from build123d import *

# Parameters (mm, degrees)
CROQUIS1_R              = 2.15
SALIENTE_EXTRUIR1_DEPTH = 320.6


with BuildPart() as part:
    # Croquis1 → Saliente-Extruir1 (new body)
    with BuildSketch(Plane.XY):
        Polygon((20, 4.95), (18.2, 6.75), (18.2, 4.4), (16.589949494, 4.4), (13.825, 7.164949494), (13.825, 12.835050506), (16.589949494, 15.6), (18.2, 15.6), (18.2, 13.25), (20, 15.05), (20, 20), (15.05, 20), (13.25, 18.2), (15.6, 18.2), (15.6, 16.589949494), (12.835050506, 13.825), (7.164949494, 13.825), (4.4, 16.589949494), (4.4, 18.2), (6.75, 18.2), (4.95, 20), (0, 20), (0, 15.05), (1.8, 13.25), (1.8, 15.6), (3.410050506, 15.6), (6.175, 12.835050506), (6.175, 7.164949494), (3.410050506, 4.4), (1.8, 4.4), (1.8, 6.75), (0, 4.95), (0, -4.95), (1.8, -6.75), (1.8, -4.4), (3.410050506, -4.4), (6.175, -7.164949494), (6.175, -12.835050506), (3.410050506, -15.6), (1.8, -15.6), (1.8, -13.25), (0, -15.05), (0, -20), (4.95, -20), (6.75, -18.2), (4.4, -18.2), (4.4, -16.589949494), (7.164949494, -13.825), (12.835050506, -13.825), (15.6, -16.589949494), (15.6, -18.2), (13.25, -18.2), (15.05, -20), (20, -20), (20, -15.05), (18.2, -13.25), (18.2, -15.6), (16.589949494, -15.6), (13.825, -12.835050506), (13.825, -7.164949494), (16.589949494, -4.4), (18.2, -4.4), (18.2, -6.75), (20, -4.95), align=None)
        with BuildLine():
            Line((1.8, -1.3), (1.8, 1.3))
            ThreePointArc((1.8, 1.3), (1.946446609, 1.653553391), (2.3, 1.8))
            Line((2.3, 1.8), (4.4, 1.8))
            Line((4.4, 1.8), (4.4, 3.410050506))
            Line((4.4, 3.410050506), (7.164949494, 6.175))
            Line((7.164949494, 6.175), (12.835050506, 6.175))
            Line((12.835050506, 6.175), (15.6, 3.410050506))
            Line((15.6, 3.410050506), (15.6, 1.8))
            Line((15.6, 1.8), (17.7, 1.8))
            ThreePointArc((17.7, 1.8), (18.053553391, 1.653553391), (18.2, 1.3))
            Line((18.2, 1.3), (18.2, -1.3))
            ThreePointArc((18.2, -1.3), (18.053553391, -1.653553391), (17.7, -1.8))
            Line((17.7, -1.8), (15.6, -1.8))
            Line((15.6, -1.8), (15.6, -3.410050506))
            Line((15.6, -3.410050506), (12.835050506, -6.175))
            Line((12.835050506, -6.175), (7.164949494, -6.175))
            Line((7.164949494, -6.175), (4.4, -3.410050506))
            Line((4.4, -3.410050506), (4.4, -1.8))
            Line((4.4, -1.8), (2.3, -1.8))
            ThreePointArc((2.3, -1.8), (1.946446609, -1.653553391), (1.8, -1.3))
        make_face(mode=Mode.SUBTRACT)
        with Locations((10, -10)):
            Circle(CROQUIS1_R, mode=Mode.SUBTRACT)
        with Locations((10, 10)):
            Circle(CROQUIS1_R, mode=Mode.SUBTRACT)
    extrude(amount=SALIENTE_EXTRUIR1_DEPTH)


solid = part.part
Build history of the part. All positions in model axes, mm. A direction names the side the tool comes from. Round coordinates to 2 decimals unless told otherwise and drop trailing zeros. One line per item, written item: value. Start each with the question number.
Q1. 3-axis set-ups, long thin cutter, end or side, ignore diameter. For faces 1 (the face through (10, -13.825, 158)), 2 (the face through (10, 13.825, 158)), 3 (the face through (13.825, 10, 158)): which of +Z, -Z, +X, -X, +Y, -Y reach the whole face in a straight line?
Q2. Cut at A-A on z = 147.5. Count the separate pieces of the cut face and the enclosed holes in it, plus the area to 3 significant figures.
Q3. Drop flat-ended pins along their axis: pin 1 Ø2 at (y, z) = (10, 174) entering from -X (3 decimals); pin 2 Ø4.5 at (y, z) = (8.5, 222.5) entering from +X; pin 3 Ø1.5 at (y, z) = (-13.5, 250) entering from +X; pin 4 Ø1.5 at (x, y) = (15, -9) entering from +Z. Give the stop position or say it passes through.
Q4. Two-plate mould, pull along Y, no slides. Class faces 4 (the face through (10, 6.175, 158)), 5 (the face through (18, 20, 158)), 6 (the face through (0, 0, 158)), 7 (the face through (10, -6.175, 158)): released by +Y, released by -Y, zero draft, split by the parting line, or undercut.
Q5. Probe line 1 along Y through (x, z) = (10.25, 304.5) (3 decimals); line 2 along Y through (x, z) = (17, 249.5); line 3 along X through (y, z) = (15.5, 158.5). List the from-to ranges inside material, lowest first.
Computed:
1. face 1: +Z, -Z, -Y
1. face 2: +Z, -Z, +Y
1. face 3: +Z, -Z, +X
2. separate pieces: 1
2. enclosed holes: 3
2. area: 292 mm²
3. pin 1: x = 6.175
3. pin 2: x = 18.7
3. pin 3: x = 19.2
3. pin 4: through
4. face 4: undercut
4. face 5: released by +Y
4. face 6: zero draft
4. face 7: undercut
5. line 1: -13.825 to -12.135, -7.865 to -6.175, 6.175 to 7.865, 12.135 to 13.825
5. line 2: -20 to -15.6, -4.4 to -1.8, 1.8 to 4.4, 15.6 to 20
5. line 3: 0 to 1.8, 3.51 to 5.49, 14.51 to 16.49, 18.2 to 20
